```python
from build123d import *

# Parameters (mm, degrees)
F0_R     = 33.02
F1_DEPTH = 3.302
F2_R     = 16.51
F3_DEPTH = 3.303
F5_D     = 7.62


with BuildPart() as f1:
    # F0 (on Top) → F1 (new body)
    with BuildSketch(Plane.XY):
        Circle(F0_R)
    extrude(amount=F1_DEPTH)

    # F2 (on face) → F3 (cut, through all)
    with BuildSketch(Plane.XY.offset(3.302)):
        Circle(F2_R)
    extrude(amount=-F3_DEPTH, mode=Mode.SUBTRACT)

    # F5 (through all)
    with Locations(Plane.XY.offset(3.302)):
        with Locations((17.691105, -17.691105), (-17.691105, -17.691105), (17.691105, 17.691105), (0, 25.019), (-17.691105, 17.691105)):
            Hole(F5_D / 2)


solid = f1.part
```
Verification items for the finished model (mm, model axes). Give positions to 0.01 mm unless a question says otherwise; leave off trailing zeros. Loops run counter-clockwise (first coordinate to the right, second up) from the corner with the lowest first, then second, coordinate; pieces in that order, holes last. Notation, with made-up numbers: M 47,47.5 L 65,47.5 A21 ccw 65,80.5 Z; hole C 10,-8 d6. An arc over 180 degrees is marked long. One line per question, with ' | ' between items.
Item 1: Section check D-D, the plane y = 20. Record the cut outline in (x, z).
Completed:
outline: M -26.27,0 L -20.72,0 L -20.72,3.3 L -26.27,3.3 Z; M -14.66,0 L 14.66,0 L 14.66,3.3 L -14.66,3.3 Z; M 20.72,0 L 26.27,0 L 26.27,3.3 L 20.72,3.3 Z
Item 2: Section check C-C, the plane z = 1.9. Record the cut outline in (x, y), plus the area to 3 significant figures.
Completed:
outline: C 0,0 d66.04; hole C -17.69,-17.69 d7.62; hole C -17.69,17.69 d7.62; hole C 0,0 d33.02; hole C 0,25.02 d7.62; hole C 17.69,-17.69 d7.62; hole C 17.69,17.69 d7.62 | area: 2,340 mm^2
Item 3: Thickness scan on line 1 (Y direction, x = 0, z = 1.25); line 2 (Y direction, x = 18.5, z = 1.7); line 3 (X direction, y = 20, z = 1.05). Record the ranges inside material, lowest first. Write a range as [from, to].
Completed:
line 1: y = [-33.02, -16.51], [16.51, 21.21], [28.83, 33.02] | line 2: y = [-27.35, -21.41], [-13.97, 13.97], [21.41, 27.35] | line 3: x = [-26.27, -20.72], [-14.66, 14.66], [20.72, 26.27]
Item 4: Depth check by flat-ended pin: P1, Ø1, axis at y = -6, z = 0.5, coming from the -X side. Enter the tip coordinate at first touch or a pass-through.
Completed:
P1: stops at x = -32.56
Item 5: Section check A-A, the plane x = 0. Record the cut outline in (y, z), plus the area to 3 significant figures.
Completed:
outline: M -33.02,0 L -16.51,0 L -16.51,3.3 L -33.02,3.3 Z; M 16.51,0 L 21.21,0 L 21.21,3.3 L 16.51,3.3 Z; M 28.83,0 L 33.02,0 L 33.02,3.3 L 28.83,3.3 Z | area: 83.9 mm^2
Item 6: Draft check along Y on faces 1 (the face through (-15, 8, 0)), 2 (the face through (31.5, 9.9, 1.6)), 3 (the face through (-14.67, 15.37, 1.63)). Enter one of: +Y half, -Y half, draft (parallel to the pull), parting line (faces both ways), or undercut.
Completed:
face 1: draft | face 2: parting line | face 3: undercut
Item 7: Section check B-B, the plane y = 1.5. Record the cut outline in (x, z), plus the area to 3 significant figures.
Completed:
outline: M -32.99,0 L -16.44,0 L -16.44,3.3 L -32.99,3.3 Z; M 16.44,0 L 32.99,0 L 32.99,3.3 L 16.44,3.3 Z | area: 109 mm^2
